Verification items for the finished model (mm, model axes). Face numbers are marked on the shaded views. A direction names the side the tool comes from. Give positions to 0.01 mm unless a question says otherwise; leave off trailing zeros. Order: outer loops, then holes, each group sorted by start corner. A loop starts at its lowest first (then second) coordinate and runs counter-clockwise, first axis right, second up. Notation, with made-up numbers: (57.5, 46) -> (112.5, 46) arc R27 cw to (112.5, 68) -> close; hole circle Ø9 at (-34, 31). An arc over 180 degrees is marked (long way). Return JSON: item names as keys, results as strings. Group by question number.
(1) Depth check by flat-ended pin: pin 1 Ø4 at (x, y) = (-5, -0.5) entering from -Z; pin 2 Ø10.5 at (x, z) = (0, 2.5) entering from -Y; pin 3 Ø1.8 at (x, z) = (0, 0) entering from -Y; pin 4 Ø5 at (x, y) = (9.5, 5) entering from +Z. Enter the tip coordinate at first touch or a pass-through.
(2) Tool access check on the marked faces 1, 2 and 3. Record the directions out of +Z, -Z, +X, -X, +Y, -Y that give a thin tool (end or side, any length) a straight path to the whole face; none if there is none.
(3) Cross-section at B-B on x = 0. Enter the section's corners in (y, z).
(4) Cross-section at D-D on x = -6. Enter the section's corners in (y, z), then the cut area to 3 significant figures.
(5) Release check for a two-part mould opening along Z. For the marked faces 4, 5 and 6 record: pulls with the +Z half, pulls with the -Z half, needs draft (parallel to the pull), parting line crosses it, or undercut.
(6) Cross-section at C-C on z = -7.5. Enter the section's corners in (x, y), then the cut area to 3 significant figures.
(7) Thickness scan on line 1 along X through (y, z) = (0.85, 0); line 2 along Y through (x, z) = (-4, -15.5); line 3 along Y through (x, z) = (6, -11). Record the ranges inside material, lowest first.
(8) Cross-section at A-A on z = 0. Enter the section's corners in (x, y), then the cut area to 3 significant figures.
from build123d import *

# Parameters (mm, degrees)
SKETCH1_R           = 17.5
BOSS_EXTRUDE1_DEPTH = 8.2
SKETCH6_R           = 12
BOSS_EXTRUDE4_DEPTH = 2
SKETCH3_R           = 13
BOSS_EXTRUDE5_DEPTH = 3.2
SKETCH7_R           = 10.8
CUT_EXTRUDE3_DEPTH  = 4
CUT_EXTRUDE4_START  = -5.2
SKETCH8_R           = 10.8
CUT_EXTRUDE4_DEPTH  = 5.2
SKETCH9_R           = 1.5
CUT_EXTRUDE5_DEPTH  = 27.071823872


with BuildPart() as part:
    # Sketch1 → Boss-Extrude1 (new body)
    with BuildSketch(Plane(origin=(0, 0, 0), x_dir=(1, 0, 0), z_dir=(0, 1, 0))):
        with Locations(Location((0, 0, 0), (0, 0, 270))):
            Circle(SKETCH1_R)
    extrude(amount=BOSS_EXTRUDE1_DEPTH)

    # Sketch6 → Boss-Extrude4 (add)
    with BuildSketch(Plane.XZ):
        with Locations(Location((0, 0, 0), (0, 0, 90))):
            Circle(SKETCH6_R)
    extrude(amount=BOSS_EXTRUDE4_DEPTH)

    # Sketch3 → Boss-Extrude5 (add)
    with BuildSketch(Plane(origin=(0, 8.2, 0), x_dir=(1, 0, 0), z_dir=(0, 1, 0))):
        with Locations(Location((0, 0, 0), (0, 0, 270))):
            Circle(SKETCH3_R)
    extrude(amount=BOSS_EXTRUDE5_DEPTH)

    # Sketch7 → Cut-Extrude3 (cut)
    with BuildSketch(Plane.XZ.offset(2)):
        with Locations(Location((0, 0, 0), (0, 0, 270))):
            Circle(SKETCH7_R)
    extrude(amount=-CUT_EXTRUDE3_DEPTH, mode=Mode.SUBTRACT)

    # Sketch8 → Cut-Extrude4 (cut)
    with BuildSketch(Plane(origin=(0, 11.4, 0), x_dir=(1, 0, 0), z_dir=(0, 1, 0)).offset(CUT_EXTRUDE4_START)):
        with Locations(Location((0, 0, 0), (0, 0, 90))):
            Circle(SKETCH8_R)
    extrude(amount=CUT_EXTRUDE4_DEPTH, mode=Mode.SUBTRACT)

    # Sketch9 → Cut-Extrude5 (cut, through all)
    with BuildSketch(Plane(origin=(0, 6.2, 0), x_dir=(1, 0, 0), z_dir=(0, 1, 0))):
        with Locations(Location((0, 0, 0), (0, 0, 270))):
            Circle(SKETCH9_R)
    extrude(amount=-CUT_EXTRUDE5_DEPTH, mode=Mode.SUBTRACT)


solid = part.part
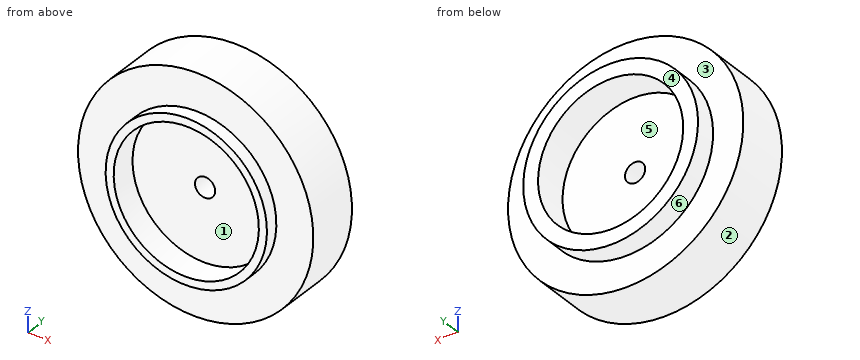
Verdict:
{
 "1": {"pin 1": "z = -17.23", "pin 2": "y = 2", "pin 3": "through", "pin 4": "z = 16.04"},
 "2": {"face 1": "-Y", "face 2": "+Y, -Y", "face 3": "+Y"},
 "3": {"outline": "(-2, -12) -> (0, -12) -> (0, -17.5) -> (8.2, -17.5) -> (8.2, -13) -> (11.4, -13) -> (11.4, -10.8) -> (6.2, -10.8) -> (6.2, -1.5) -> (2, -1.5) -> (2, -10.8) -> (-2, -10.8) -> close; (-2, 10.8) -> (2, 10.8) -> (2, 1.5) -> (6.2, 1.5) -> (6.2, 10.8) -> (11.4, 10.8) -> (11.4, 13) -> (8.2, 13) -> (8.2, 17.5) -> (0, 17.5) -> (0, 12) -> (-2, 12) -> close"},
 "4": {"outline": "(-2, -10.39) -> (0, -10.39) -> (0, -16.44) -> (8.2, -16.44) -> (8.2, -11.53) -> (11.4, -11.53) -> (11.4, -8.98) -> (6.2, -8.98) -> (6.2, 8.98) -> (11.4, 8.98) -> (11.4, 11.53) -> (8.2, 11.53) -> (8.2, 16.44) -> (0, 16.44) -> (0, 10.39) -> (-2, 10.39) -> (-2, 8.98) -> (2, 8.98) -> (2, -8.98) -> (-2, -8.98) -> close", "area": "220 mm²"},
 "5": {"face 4": "needs draft", "face 5": "undercut", "face 6": "parting line crosses it"},
 "6": {"outline": "(-15.81, 0) -> (-9.37, 0) -> (-9.37, -2) -> (-7.77, -2) -> (-7.77, 2) -> (7.77, 2) -> (7.77, -2) -> (9.37, -2) -> (9.37, 0) -> (15.81, 0) -> (15.81, 8.2) -> (10.62, 8.2) -> (10.62, 11.4) -> (7.77, 11.4) -> (7.77, 6.2) -> (-7.77, 6.2) -> (-7.77, 11.4) -> (-10.62, 11.4) -> (-10.62, 8.2) -> (-15.81, 8.2) -> close", "area": "222 mm²"},
 "7": {"line 1": "-17.5 to -10.8, 10.8 to 17.5", "line 2": "0 to 8.2", "line 3": "0 to 11.4"},
 "8": {"outline": "(-17.5, 0) -> (-12, 0) -> (-12, -2) -> (-10.8, -2) -> (-10.8, 2) -> (-1.5, 2) -> (-1.5, 6.2) -> (-10.8, 6.2) -> (-10.8, 11.4) -> (-13, 11.4) -> (-13, 8.2) -> (-17.5, 8.2) -> close; (1.5, 2) -> (10.8, 2) -> (10.8, -2) -> (12, -2) -> (12, 0) -> (17.5, 0) -> (17.5, 8.2) -> (13, 8.2) -> (13, 11.4) -> (10.8, 11.4) -> (10.8, 6.2) -> (1.5, 6.2) -> close", "area": "207 mm²"}
}
